The model under review builds one solid part; all positions refer to its coordinate system, in mm. Round coordinates to 2 decimals unless told otherwise and drop trailing zeros. Loops run counter-clockwise (first coordinate to the right, second up) from the corner with the lowest first, then second, coordinate; pieces in that order, holes last. Notation, with made-up numbers: M -12.75,-16.75 L 16.25,-16.75 A26 cw 16.25,0.25 Z; hole C 54.25,63.5 d5. An arc over 180 degrees is marked long. One line per question, with ' | ' between items.
from build123d import *

# Parameters (mm, degrees)
SKETCH1_R               = 25.4
BOSS_EXTRUDE1_DEPTH     = 50.8
SKETCH3_R               = 57.740846599
CUT_EXTRUDE1_DEPTH      = 124.114128787
SKETCH4_RX              = 6.35
SKETCH4_RY              = 5.08
CUT_EXTRUDE2_DEPTH      = 152.575785835
CUT_EXTRUDE3_REACH      = 157.303
CUT_EXTRUDE3_END_RADIUS = 25.4
SKETCH6_R               = 5.08


with BuildPart() as part:
    # Sketch1 → Boss-Extrude1 (new body)
    with BuildSketch(Plane(origin=(0, 0, 0), x_dir=(1, 0, 0), z_dir=(0, 1, 0))):
        with BuildLine():
            Line((-69.85, -38.1), (31.75, -38.1))
            ThreePointArc((31.75, -38.1), (58.690768363, -26.940768363), (69.85, 0))
            Line((69.85, 0), (69.85, 38.1))
            Line((69.85, 38.1), (-69.85, 38.1))
            Line((-69.85, 38.1), (-69.85, -38.1))
        make_face()
        with Locations(Location((31.75, 0, 0), (0, 0, 270))):
            Circle(SKETCH1_R, mode=Mode.SUBTRACT)
    extrude(amount=BOSS_EXTRUDE1_DEPTH)

    # Sketch3 → Cut-Extrude1 (cut, through all)
    with BuildSketch(Plane(origin=(20.144827586, 30.217241379, 40.289655172), x_dir=(0.928476690885259, -0.22283440581246322, -0.2971125410832833), z_dir=(0.3713906763541046, 0.5570860145311567, 0.7427813527082063))):
        with Locations((6.839159305, 17.78)):
            Circle(SKETCH3_R)
    extrude(amount=CUT_EXTRUDE1_DEPTH, mode=Mode.SUBTRACT)

    # Sketch4 → Cut-Extrude2 (cut, through all)
    with BuildSketch(Plane(origin=(66.003779532, 55.383747061, 0), x_dir=(0, 0, -1), z_dir=(0.7660444431189792, 0.6427876096865379, 0))):
        with Locations((-24.13, 71.113772247)):
            Ellipse(SKETCH4_RX, SKETCH4_RY)
        with Locations((24.13, 71.113772247)):
            Ellipse(SKETCH4_RX, SKETCH4_RY)
    extrude(amount=-CUT_EXTRUDE2_DEPTH, mode=Mode.SUBTRACT)

    # Cut-Extrude3: up to this cylinder (the profile starts outside it)
    cut_extrude3_end = Plane(origin=(31.75, 58.963403, 0), z_dir=(0, -1, 0)) * Cylinder(CUT_EXTRUDE3_END_RADIUS, 366.406, mode=Mode.PRIVATE)
    # Sketch6 → Cut-Extrude3 (cut, up to the surface)
    with BuildSketch(Plane(origin=(-78.005907462, 28.391828413, 0), x_dir=(0, 0, 1), z_dir=(-0.9396926207859093, 0.34202014332566605, 0)), mode=Mode.PRIVATE) as cut_extrude3_sk1:
        with Locations(Location((0, 32.533589765, 0), (0, 0, 270))):
            Circle(SKETCH6_R)
    cut_extrude3_tool1 = extrude(cut_extrude3_sk1.sketch, amount=-CUT_EXTRUDE3_REACH, mode=Mode.PRIVATE) - cut_extrude3_end
    add(cut_extrude3_tool1.solids().sort_by_distance((-66.878764, 58.963403, 0))[0], mode=Mode.SUBTRACT)


solid = part.part
1) Insertion check: P1, Ø5, axis at x = 54, z = 27, coming from the +Y side; P2, Ø10, axis at x = 39, y = 23.5, coming from the +Z side; P3, Ø6, axis at x = 22.5, z = -20.5, coming from the +Y side; P4, Ø8, axis at y = 27.5, z = 17, coming from the +X side. Each pin has a flat end and moves straight along its axis. Give the tip position at first contact, or say it passes through.
Output values:
P1: stops at y = 29.09 | P2: stops at z = 38.03 | P3: stops at y = 50.8 | P4: stops at x = 67.56
2) Mouldability with a two-part tool opening along Z and no side actions: class faces 1 (the flat face through (-20, 25, 38.1)), 2 (the cylindrical face through (16.294, 25.044, -20.157)), 3 (the cylindrical face through (-19.561, 36.585, 1.526)), 4 (the flat face through (-69.85, 25, -1)) as +Z half, -Z half, draft (parallel to the pull), parting line (faces both ways), or undercut.
Output values:
face 1: +Z half | face 2: undercut | face 3: undercut | face 4: draft
3) Add section B-B on z = -1.5. State the section outline as (x, y) points.
Output values:
outline: M -69.85,0 L 6.39,0 L 6.39,27.13 L -58.64,50.8 L -69.85,50.8 Z; M -30.26,50.8 L 6.39,37.46 L 6.39,50.8 Z; M 57.11,0 L 69.85,0 L 69.85,50.8 L 57.11,50.8 Z
4) For line 1 (X direction, y = 24.5, z = 0); line 2 (Z direction, x = 31.75, y = 11); line 3 (Y direction, x = 1, z = 0), list the stretches that pass through material, from the lowest coordinate up.
Output values:
line 1: x = -69.85 to 6.35, 57.15 to 69.85 | line 2: z = -38.1 to -25.4, 25.4 to 38.1 | line 3: y = 0 to 28.85, 39.66 to 50.8
5) Add section A-A on x = 27.5. State the section outline as (y, z) points.
Output values:
outline: M 0,-38.1 L 50.8,-38.1 L 50.8,-25.04 L 0,-25.04 Z; M 0,25.04 L 45.64,25.04 L 28.23,38.1 L 0,38.1 Z
6) Add section C-C on z = -24. State how many separate pieces and enclosed holes the cut face has, then the cut area to 3 significant figures.
Output values:
separate pieces: 3 | enclosed holes: 0 | area: 5,990 mm²
